```python
from build123d import *

# Parameters (mm, degrees)
SKETCH_1_W          = 800
SKETCH_1_H          = 55
SKETCH_1_R          = 16.5
EXTRUDE_1_DEPTH     = 200
SKETCH_2_R          = 16.5
CUT_EXTRUDE_1_DEPTH = 827.453265466
FILLET_1_R          = 27.5


with BuildPart() as part:
    # 草图1 → 凸台-拉伸1 (new body)
    with BuildSketch(Plane.XY):
        with Locations((400, 27.5)):
            Rectangle(SKETCH_1_W, SKETCH_1_H)
        with Locations((300, 27.5)):
            Circle(SKETCH_1_R, mode=Mode.SUBTRACT)
        with Locations((500, 27.5)):
            Circle(SKETCH_1_R, mode=Mode.SUBTRACT)
    extrude(amount=EXTRUDE_1_DEPTH)

    # 草图2 → 切除-拉伸1 (cut, through all)
    with BuildSketch(Plane.XY.offset(200)):
        with Locations((759.807621135, 27.5)):
            Circle(SKETCH_2_R)
        with Locations((40.192378865, 27.5)):
            Circle(SKETCH_2_R)
    extrude(amount=-CUT_EXTRUDE_1_DEPTH, mode=Mode.SUBTRACT)

    # 圆角1
    fillet_1_edges = [part.edges().sort_by_distance(p)[0] for p in [
        (0, 0, 100),
        (0, 55, 100),
        (800, 0, 100),
        (800, 55, 100),
    ]]
    fillet(fillet_1_edges, radius=FILLET_1_R - 0.0001)  # a hair under: the kernel refuses the full size


solid = part.part
```
The listing builds one solid part. Answer for the finished solid, in the listing's coordinates (mm). Coordinates: 2 decimals unless noted, no trailing zeros. Loops run counter-clockwise (first coordinate to the right, second up) from the corner with the lowest first, then second, coordinate; pieces in that order, holes last. Notation, with made-up numbers: (-15.75, 4.5) - (16.25, 4.5) arc R19 ccw to (16.25, 27.5) - close; hole circle Ø1 at (2.25, 20.25). An arc over 180 degrees is marked (long way). Use a Markdown table: item, result. Add a question column.
1) The part is cut by section B-B, the plane z = 73. State how many separate pieces and enclosed holes the cut face has, and give its area (3 significant figures).
2) The part is cut by section C-C, the plane x = 494. Give the vertices of the cut face in (y, z), and give its area (3 significant figures).
3) The mould has two halves that part along X. Classify faces 1 (the flat face through (395, 55, 99)), 2 (the cylindrical face through (27.1, 17.46, 101.4)), 3 (the cylindrical face through (515.738, 32.456, 98.6)), 4 (the cylindrical face through (7.84, 46.73, 101.4)): released by +X, released by -X, zero draft, split by the parting line, or undercut.
4) Given pin 1 (1 mm diameter, centred on y = 37.5, z = 37, fed in from -X); pin 2 (3 mm diameter, centred on y = 31, z = 71, fed in from -X); pin 3 (6 mm diameter, centred on y = 37.5, z = 77.5, fed in from +X), each flat-ended and moving along its own axis, determine where each tip first touches the part or whether it passes through.
5) The part is cut by section A-A, the plane x = 300. Give the vertices of the cut face in (y, z), and give its area (3 significant figures).
6) Find the intervals of material crossed by line 1 (X direction, y = 26.5, z = 65); line 2 (Y direction, x = 500, z = 86); line 3 (X direction, y = 35, z = 186.5), in increasing order.
Here are the results:
| question | item | result |
|---|---|---|
| 1 | separate pieces | 1 |
| 1 | enclosed holes | 4 |
| 1 | area | 39,900 mm^2 |
| 2 | outline | (0, 0) - (12.13, 0) - (12.13, 200) - (0, 200) - close; (42.87, 0) - (55, 0) - (55, 200) - (42.87, 200) - close |
| 2 | area | 4,850 mm^2 |
| 3 | face 1 | zero draft |
| 3 | face 2 | undercut |
| 3 | face 3 | undercut |
| 3 | face 4 | released by -X |
| 4 | pin 1 | stops at x = 1.69 |
| 4 | pin 2 | stops at x = 0.07 |
| 4 | pin 3 | stops at x = 799.09 |
| 5 | outline | (0, 0) - (11, 0) - (11, 200) - (0, 200) - close; (44, 0) - (55, 0) - (55, 200) - (44, 200) - close |
| 5 | area | 4,400 mm^2 |
| 6 | line 1 | x = 0.02 to 23.72, 56.66 to 283.53, 316.47 to 483.53, 516.47 to 743.34, 776.28 to 799.98 |
| 6 | line 2 | y = 0 to 11, 44 to 55 |
| 6 | line 3 | x = 1.04 to 25.5, 54.89 to 285.3, 314.7 to 485.3, 514.7 to 745.11, 774.5 to 798.96 |
